Geometry: final body of the model. Coordinates: model frame, mm. A direction names the side the tool comes from. Give positions to 0.01 mm unless a question says otherwise; leave off trailing zeros. Write each loop counter-clockwise with the first axis right and the second up, starting at its lowest first coordinate (ties: lowest second). Pieces come first, ordered by that corner, then holes.
Q1. Line query: L1, parallel to Y at x = 2, z = -6.25; L2, parallel to Z at x = 4, y = 1.3; L3, parallel to Y at x = 6.25, z = -0.5. Output: solid intervals per line, ascending.
Q2. Cut plane D-D on x = 5.25. Return the cut outline in (y, z).
Q3. Cut plane C-C on y = 0.7. Return the cut outline in (x, z).
Q4. Cut plane A-A on z = -5.5. Return the cut outline in (x, y).
Q5. Reachability of faces 1 (the face through (3.9, 0.5, -8.8)), 2 (the face through (2.4, 2.48, -5.57)), 3 (the face through (3.8, 0.5, -0.5)) from +Z, -Z, +X, -X, +Y, -Y: full face, straight path, thin tool, end or side. Return the list, or none.
Q6. Cut plane B-B on x = 3.9. Return the cut outline in (y, z), plus the area to 3 significant figures.
Q7. Pin query (flat end, axial travel): pin 1 (1 mm diameter, centred on x = 4.5, y = 3, fed in from +Z); pin 2 (1.5 mm diameter, centred on y = 2.5, z = -5.5, fed in from +X); pin 3 (0.6 mm diameter, centred on x = 3.5, y = 1, fed in from +Z). Return the tip coordinate at first contact, or that it passes through.
```python
from build123d import *

# Parameters (mm, degrees)
BOSS_EXTRUDE1_DEPTH = 1
SKETCH2_R           = 1.5
BOSS_EXTRUDE2_DEPTH = 3
SKETCH3_W           = 7.8
SKETCH3_H           = 1
CUT_EXTRUDE1_DEPTH  = 0.5


with BuildPart() as part:
    # Sketch1 → Boss-Extrude1 (new body)
    with BuildSketch(Plane(origin=(0, 0, 0), x_dir=(1, 0, 0), z_dir=(0, 1, 0))):
        with BuildLine():
            Line((0, 0), (7.8, 0))
            Line((7.8, 0), (7.8, 5.8))
            ThreePointArc((7.8, 5.8), (6.921320344, 7.921320344), (4.8, 8.8))
            Line((4.8, 8.8), (3, 8.8))
            ThreePointArc((3, 8.8), (0.878679656, 7.921320344), (0, 5.8))
            Line((0, 5.8), (0, 0))
        make_face()
    extrude(amount=BOSS_EXTRUDE1_DEPTH)

    # Sketch2 → Boss-Extrude2 (add)
    with BuildSketch(Plane(origin=(0, 1, 0), x_dir=(1, 0, 0), z_dir=(0, 1, 0))):
        with Locations((3.9, 5.5)):
            Circle(SKETCH2_R)
    extrude(amount=BOSS_EXTRUDE2_DEPTH)

    # Sketch3 → Cut-Extrude1 (cut)
    with BuildSketch(Plane(origin=(0, 1, 0), x_dir=(1, 0, 0), z_dir=(0, 1, 0))):
        with Locations((3.9, 0.5)):
            Rectangle(SKETCH3_W, SKETCH3_H)
    extrude(amount=-CUT_EXTRUDE1_DEPTH, mode=Mode.SUBTRACT)


solid = part.part
```
Data:
1. L1: y = 0 to 1
1. L2: z = -7 to -4
1. L3: y = 0 to 0.5
2. outline: (0, -8.77) - (1, -8.77) - (1, -6.15) - (4, -6.15) - (4, -4.85) - (1, -4.85) - (1, -1) - (0.5, -1) - (0.5, 0) - (0, 0) - close
3. outline: (0, -5.8) arc R3 ccw to (3, -8.8) - (4.8, -8.8) arc R3 ccw to (7.8, -5.8) - (7.8, -1) - (0, -1) - close
4. outline: (0, 0) - (7.8, 0) - (7.8, 1) - (5.4, 1) - (5.4, 4) - (2.4, 4) - (2.4, 1) - (0, 1) - close
5. face 1: -Z, +X, -X, +Y, -Y
5. face 2: +Y
5. face 3: +Z, +X, -X, +Y
6. outline: (0, -8.8) - (1, -8.8) - (1, -7) - (4, -7) - (4, -4) - (1, -4) - (1, -1) - (0.5, -1) - (0.5, 0) - (0, 0) - close
6. area: 17.3 mm2
7. pin 1: stops at z = -4
7. pin 2: stops at x = 5.4
7. pin 3: stops at z = -1
